from build123d import *

# Parameters (mm, degrees)
SM_BASE_FLANGE_1_DEPTH  = 29.75
CUT_EXTRUDE_START       = -2
CUT_EXTRUDE_1_OUTLINE_W = 40
CUT_EXTRUDE_1_OUTLINE_H = 22
CUT_EXTRUDE_1_OUTLINE_R = 2.25
CUT_EXTRUDE_1_DEPTH     = 2
SKETCH_7_R              = 2
SKETCH_7_W              = 40
SKETCH_7_H              = 10
CUT_EXTRUDE_4_DEPTH     = 44.070436497
FILLET_1_R              = 1


# Read off the part's stored shape, not the designer's step: 切除-拉伸1
# Sheet-metal steps are written as plain solids
with BuildPart() as part:
    # Sketch 1 → 基体-法兰1 (new, symmetric)
    with BuildSketch(Plane.ZY):
        with BuildLine():
            Line((-20, 0), (-1, 0))
            ThreePointArc((-1, 0), (-0.292893219, -0.292893219), (0, -1))
            Line((0, -1), (0, -23))
            Line((0, -23), (1, -23))
            Line((1, -23), (1, -1))
            ThreePointArc((1, -1), (0.414213562, 0.414213562), (-1, 1))
            Line((-1, 1), (-20, 1))
            Line((-20, 1), (-20, 0))
        make_face()
    extrude(amount=SM_BASE_FLANGE_1_DEPTH, both=True)

    # 切除-拉伸1 outline → 切除-拉伸1 (cut)
    with BuildSketch(Plane(origin=(0, 1, 0), x_dir=(1, 0, 0), z_dir=(0, 1, 0)).offset(CUT_EXTRUDE_START)):
        with Locations((0, 9)):
            Rectangle(CUT_EXTRUDE_1_OUTLINE_W, CUT_EXTRUDE_1_OUTLINE_H)
        with Locations((-24.75, 15)):
            Circle(CUT_EXTRUDE_1_OUTLINE_R)
        with Locations((24.75, 15)):
            Circle(CUT_EXTRUDE_1_OUTLINE_R)
        with Locations((24.75, 5)):
            Circle(CUT_EXTRUDE_1_OUTLINE_R)
        with Locations((-24.75, 5)):
            Circle(CUT_EXTRUDE_1_OUTLINE_R)
    extrude(amount=CUT_EXTRUDE_1_DEPTH, mode=Mode.SUBTRACT)

    # 草图7 → 切除-拉伸4 (cut, through all)
    with BuildSketch(Plane.XY.offset(1)):
        with Locations((-24.75, -6)):
            Circle(SKETCH_7_R)
        with Locations((-24.75, -18)):
            Circle(SKETCH_7_R)
        with Locations((24.75, -18)):
            Circle(SKETCH_7_R)
        with Locations((24.75, -6)):
            Circle(SKETCH_7_R)
        with Locations((0, -12)):
            Rectangle(SKETCH_7_W, SKETCH_7_H)
    extrude(amount=-CUT_EXTRUDE_4_DEPTH, mode=Mode.SUBTRACT)

    # 圆角1
    fillet_1_edges = [part.edges().sort_by_distance(p)[0] for p in [
        (-20, -17, 0.5),
        (-20, -7, 0.5),
        (20, -7, 0.5),
        (20, -17, 0.5),
        (-29.75, 0.5, -20),
        (20, 0.5, -20),
        (-20, 0.5, -20),
        (-29.75, -23, 0.5),
        (29.75, 0.5, -20),
        (29.75, -23, 0.5),
    ]]
    fillet(fillet_1_edges, radius=FILLET_1_R)


solid = part.part
Geometry check sheet. Reference: the model listing, model coordinates, mm. A direction names the side the tool comes from. Round coordinates to 2 decimals unless told otherwise and drop trailing zeros. Loops run counter-clockwise (first coordinate to the right, second up) from the corner with the lowest first, then second, coordinate; pieces in that order, holes last.
Item 1: Cross-section at B-B on x = -24.75. Record the boundary of the cut face in (y, z), then the cut area to 3 significant figures.
Item 2: Access from +Z, -Z, +X, -X, +Y, -Y to the whole of each face (thin tool, end or side, straight path). Record for faces 5 (the flat face through (-7, -5, 0)), 6 (the cylindrical face through (24.81, 0.4, 0.43)), 7 (the flat face through (-20, 0.4, -8.9)).
Item 3: Gauge pin test, flat ends, axial feed: pin 1 (12 mm diameter, centred on x = 16.5, y = -10, fed in from -Z); pin 2 (8 mm diameter, centred on x = 15.5, z = -3.5, fed in from +Y); pin 3 (10.5 mm diameter, centred on x = 24, z = -13, fed in from -Y). Record the tip position at first contact, or that the pin passes through.
Item 4: Cross-section at C-C on z = -15. Record the boundary of the cut face in (x, y), then the cut area to 3 significant figures.
Item 5: Cross-section at A-A on z = -10. Record the boundary of the cut face in (x, y), then the cut area to 3 significant figures.
Item 6: Thickness scan on line 1 (X direction, y = 0.7, z = -15); line 2 (Y direction, x = -24.75, z = 0.55); line 3 (Y direction, x = 27, z = -16.25). Record the ranges inside material, lowest first.
Item 7: Cross-section at D-D on y = -18. Record the boundary of the cut face in (x, z).
Item 8: Mould release check, pull along Z, two halves, no side actions. Record for faces 1 (the cylindrical face through (-24.94, 0.4, 0.43)), 2 (the cylindrical face through (22.752, -5.912, 0.507)), 3 (the cylindrical face through (-23.712, 0.493, -13.004)), 4 (the cylindrical face through (25.788, 0.493, -13.004)): pulls with the +Z half, pulls with the -Z half, needs draft (parallel to the pull), parting line crosses it, or undercut.
Answer sheet:
1. outline: (-23, 0) - (-20, 0) - (-20, 1) - (-23, 1) - close; (-16, 0) - (-8, 0) - (-8, 1) - (-16, 1) - close; (-4, 0) - (-1, 0) arc R1 cw to (0, -1) - (0, -2.75) - (1, -2.75) - (1, -1) arc R2 ccw to (-1, 1) - (-4, 1) - close; (0, -20) - (1, -20) - (1, -17.25) - (0, -17.25) - close; (0, -12.75) - (1, -12.75) - (1, -7.25) - (0, -7.25) - close
1. area: 26.4 mm2
2. face 5: -Z, +X, -X, -Y
2. face 6: +Z, +X, -X, +Y
2. face 7: +Z, -Z, +Y
3. pin 1: stops at z = 0
3. pin 2: stops at y = -1
3. pin 3: stops at y = 0
4. outline: (-29.75, 0) - (-27, 0) - (-27, 1) - (-29.75, 1) - close; (-22.5, 0) - (-20, 0) - (-20, 1) - (-22.5, 1) - close; (20, 0) - (22.5, 0) - (22.5, 1) - (20, 1) - close; (27, 0) - (29.75, 0) - (29.75, 1) - (27, 1) - close
4. area: 10.5 mm2
5. outline: (-29.75, 0) - (-20, 0) - (-20, 1) - (-29.75, 1) - close; (20, 0) - (29.75, 0) - (29.75, 1) - (20, 1) - close
5. area: 19.5 mm2
6. line 1: x = -29.75 to -27, -22.5 to -20, 20 to 22.5, 27 to 29.75
6. line 2: y = -23 to -20, -16 to -8, -4 to 0.26
6. line 3: y = 0 to 1
7. outline: (-29.75, 0) - (-26.75, 0) - (-26.75, 1) - (-29.75, 1) - close; (-22.75, 0) - (22.75, 0) - (22.75, 1) - (-22.75, 1) - close; (26.75, 0) - (29.75, 0) - (29.75, 1) - (26.75, 1) - close
8. face 1: pulls with the +Z half
8. face 2: needs draft
8. face 3: undercut
8. face 4: undercut
